CAD build for the part. Positions are in the model's coordinates, mm. Face numbers are marked on the shaded views. A direction names the side the tool comes from. Round coordinates to 2 decimals unless told otherwise and drop trailing zeros. Loops run counter-clockwise (first coordinate to the right, second up) from the corner with the lowest first, then second, coordinate; pieces in that order, holes last. Notation, with made-up numbers: (-37.75, 0.25) - (-27.75, 0.25) arc R16 ccw to (-27.75, 19.25) - close; hole circle Ø5 at (-33, -3.75). An arc over 180 degrees is marked (long way). Use one line per item in the form item = value.
Autodesk Inventor part; units mm, degrees
ref_plane "YZ Plane" through (0, 0, 0) normal (1, 0, 0) x (0, 1, 0)
ref_plane "XZ Plane" through (0, 0, 0) normal (0, 1, 0) x (-1, 0, 0)
ref_plane "XY Plane" through (0, 0, 0) normal (0, 0, 1) x (1, 0, 0)
sketch "Sketch1" plane through (0, 0, 0) normal (0, 1, 0) x (-1, 0, 0)
  line L0 (0, 0) -> (16, 0)
  line L1 (16, 0) -> (16, -120)
  line L2 (16, -120) -> (0, -120)
  line L3 (0, -120) -> (0, 0)
  dimension "d0" = 120
  dimension "d1" = 16
extrude "Extrusion" add sketch "Sketch1" along normal blind 16
sketch "Sketch2" plane through (0, 16, 0) normal (0, 1, 0) x (1, 0, 0)
  line L0 (0, 120) -> (-16, 120)
  line L1 (-16, 120) -> (-16, 0)
  line L2 (-16, 0) -> (0, 0)
  line L3 (0, 0) -> (0, 120)
  line L4 (-16, 120) -> (-16, 0)
  line L5 (-16, 0) -> (0, 0)
  line L6 (0, 0) -> (0, 26.5)
  line L7 (0, 26.5) -> (-16, 26.5)
  line L8 (-16, 26.5) -> (-16, 0)
  line L9 (0, 0) -> (0, 120)
  line L10 (-16, 120) -> (0, 120)
  line L11 (0, 120) -> (0, 93.5)
  line L12 (0, 93.5) -> (-16, 93.5)
  line L13 (-16, 93.5) -> (-16, 120)
  point P0 (-8, 26.5)
  point P1 (-16, 93.5)
  point P2 (-16, 26.5)
  dimension "d4" = 26.5
  dimension "d5" = 26.5
extrude "Extrusion2" cut sketch "Sketch2" against normal blind 8 contours L3 L12 L1 L0 | L3 L2 L1 L7
sketch "Sketch3" plane through (0, 0, 0) normal (0, -1, 0) x (1, 0, 0)
  line L0 (0, -120) -> (-16, -120)
  line L1 (0, 0) -> (0, -120)
  line L2 (-16, 0) -> (0, 0)
  line L3 (-16, -120) -> (-16, 0)
  circle A0 centre (-8, -6) radius 1.55
  line L4 (0, -26.5) -> (0, -93.5) construction
  line L5 (0, -60) -> (-16, -60) construction
  line L6 (-16, -120) -> (-16, 0) construction
  circle A1 centre (-8, -18) radius 1.55
  circle A2 centre (-8, -114) radius 1.55
  circle A3 centre (-8, -102) radius 1.55
  dimension "d8" = 3.1
  dimension "d9" = 8
  dimension "d10" = 6
  dimension "d11" = 12
extrude "Extrusion3" cut sketch "Sketch3" against normal through all contours A0 | A1 | A2 | A3
sketch "Sketch4" plane through (0, 0, 0) normal (0, -1, 0) x (1, 0, 0)
  circle A0 centre (-8, -6) radius 1.55
  circle A1 centre (-8, -114) radius 1.55
  circle A2 centre (-8, -18) radius 1.55
  circle A3 centre (-8, -102) radius 1.55
  line L0 (0, -120) -> (-16, -120)
  line L1 (0, 0) -> (0, -120)
  line L2 (-16, 0) -> (0, 0)
  line L3 (-16, -120) -> (-16, 0)
  circle A4 centre (-8, -6) radius 1.55
  line L4 (-8, -2.7668) -> (-5.2, -4.3834)
  line L5 (-5.2, -4.3834) -> (-5.2, -7.6166)
  line L6 (-5.2, -7.6166) -> (-8, -9.2332)
  line L7 (-8, -9.2332) -> (-10.8, -7.6166)
  line L8 (-10.8, -7.6166) -> (-10.8, -4.3834)
  line L9 (-10.8, -4.3834) -> (-8, -2.7668)
  line L10 (-8, -14.7668) -> (-5.2, -16.3834)
  line L11 (-5.2, -16.3834) -> (-5.2, -19.6166)
  line L12 (-5.2, -19.6166) -> (-8, -21.2332)
  line L13 (-8, -21.2332) -> (-10.8, -19.6166)
  line L14 (-10.8, -19.6166) -> (-10.8, -16.3834)
  line L15 (-10.8, -16.3834) -> (-8, -14.7668)
  line L16 (-8, -98.7668) -> (-5.2, -100.3834)
  line L17 (-5.2, -100.3834) -> (-5.2, -103.6166)
  line L18 (-5.2, -103.6166) -> (-8, -105.2332)
  line L19 (-8, -105.2332) -> (-10.8, -103.6166)
  line L20 (-10.8, -103.6166) -> (-10.8, -100.3834)
  line L21 (-10.8, -100.3834) -> (-8, -98.7668)
  line L22 (-8, -110.7668) -> (-5.2, -112.3834)
  line L23 (-5.2, -112.3834) -> (-5.2, -115.6166)
  line L24 (-5.2, -115.6166) -> (-8, -117.2332)
  line L25 (-8, -117.2332) -> (-10.8, -115.6166)
  line L26 (-10.8, -115.6166) -> (-10.8, -112.3834)
  line L27 (-10.8, -112.3834) -> (-8, -110.7668)
  dimension "d14" = 5.6
  dimension "d15" = 5.6
  dimension "d16" = 5.6
  dimension "d17" = 5.6
extrude "Extrusion4" cut sketch "Sketch4" against normal blind 2.5 contours L4 L5 L6 L7 L8 L9 | L10 L11 L12 L13 L14 L15 | L16 L17 L18 L19 L20 L21 | L22 L23 L24 L25 L26 L27
properties part number "A_base"
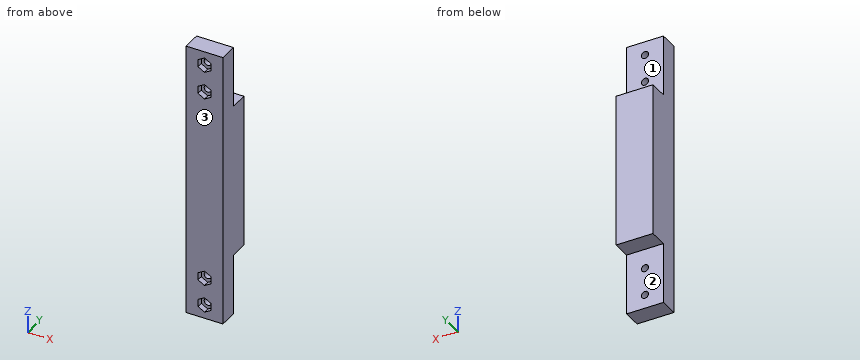
1) Slice it at B-B (y = 6.5). Write the cut outline in (x, z), plus the area to 3 significant figures.
Report:
outline = (-16, -120) - (0, -120) - (0, 0) - (-16, 0) - close; hole circle Ø3.1 at (-8, -114); hole circle Ø3.1 at (-8, -102); hole circle Ø3.1 at (-8, -18); hole circle Ø3.1 at (-8, -6)
area = 1,890 mm^2
2) Drill centre lines: probe 1 along Z at (x, y) = (-8, 5.85); probe 2 along X at (y, z) = (4.5, -102); probe 3 along Y at (x, z) = (-2.5, -22). Where is each one in solid material? Low to high.
Report:
probe_1 = -120 to -115.55, -112.45 to -103.55, -100.45 to -19.55, -16.45 to -7.55, -4.45 to 0
probe_2 = -16 to -9.55, -6.45 to 0
probe_3 = 0 to 8
3) Tool access for the marked faces 1, 2 and 3: list every direction of +Z, -Z, +X, -X, +Y, -Y with a clear straight run to the whole face (end or side of a thin tool).
Report:
face_1 = +Z, +X, -X, +Y
face_2 = -Z, +X, -X, +Y
face_3 = +Z, -Z, +X, -X, -Y
4) Flat gauge pins, fed straight in: pin 1 (6.5 mm diameter, centred on x = -7.5, y = 13.5, fed in from -Z); pin 2 (2.5 mm diameter, centred on x = -8, z = -102, fed in from -Y); pin 3 (3.5 mm diameter, centred on x = -8, z = -114, fed in from -Y); pin 4 (4 mm diameter, centred on x = -10, y = 12, fed in from +Z). Where does each tip first touch, or does it go through?
Report:
pin_1 = -93.5
pin_2 = through
pin_3 = 2.5
pin_4 = -26.5
5) Slice it at D-D (y = 14). Write the cut outline in (x, z).
Report:
outline = (-16, -93.5) - (0, -93.5) - (0, -26.5) - (-16, -26.5) - close
6) Slice it at A-A (z = -18). Write the cut outline in (x, y).
Report:
outline = (-16, 0) - (-10.8, 0) - (-10.8, 2.5) - (-9.55, 2.5) - (-9.55, 8) - (-16, 8) - close; (-6.45, 2.5) - (-5.2, 2.5) - (-5.2, 0) - (0, 0) - (0, 8) - (-6.45, 8) - close
7) Slice it at C-C (x = -4). Write the cut outline in (y, z), plus the area to 3 significant figures.
Report:
outline = (0, -120) - (8, -120) - (8, -93.5) - (16, -93.5) - (16, -26.5) - (8, -26.5) - (8, 0) - (0, 0) - close
area = 1,500 mm^2
